Here's how the part is built. I have some questions about the finished solid (model axes, mm). A direction names the side the tool comes from. Coordinates: 2 decimals unless noted, no trailing zeros. Order: outer loops, then holes, each group sorted by start corner. A loop starts at its lowest first (then second) coordinate and runs counter-clockwise, first axis right, second up. Notation, with made-up numbers: M -29,34.5 L 29,34.5 A22 ccw 29,61.5 Z; hole C 53.25,75 d8. An arc over 180 degrees is marked long. Answer as CSV lines item,"result". Start each with the question number.
```python
from build123d import *

# Parameters (mm, degrees)
SKETCH1_W           = 82.042
SKETCH1_H           = 56.388
SKETCH1_R           = 1.651
BOSS_EXTRUDE1_DEPTH = 2.54
SKETCH2_W           = 19.05
SKETCH2_H           = 2.7432
SKETCH2_W_2         = 2.7432
SKETCH2_H_2         = 19.05
BOSS_EXTRUDE2_DEPTH = 2.54
SKETCH3_W           = 30.48
SKETCH3_H           = 9.525
CUT_EXTRUDE1_DEPTH  = 3.54


with BuildPart() as part:
    # Sketch1 → Boss-Extrude1 (new body)
    with BuildSketch(Plane(origin=(0, 0, 0), x_dir=(1, 0, 0), z_dir=(0, 1, 0))):
        Rectangle(SKETCH1_W, SKETCH1_H)
        with Locations((-34.671, 21.844)):
            Circle(SKETCH1_R, mode=Mode.SUBTRACT)
        with Locations((-34.671, -21.844)):
            Circle(SKETCH1_R, mode=Mode.SUBTRACT)
        with Locations((34.671, -21.844)):
            Circle(SKETCH1_R, mode=Mode.SUBTRACT)
        with Locations((34.671, 21.844)):
            Circle(SKETCH1_R, mode=Mode.SUBTRACT)
    extrude(amount=BOSS_EXTRUDE1_DEPTH)

    # Sketch2 → Boss-Extrude2 (add)
    with BuildSketch(Plane(origin=(0, 2.54, 0), x_dir=(1, 0, 0), z_dir=(0, 1, 0))):
        with Locations((0, 29.5656)):
            Rectangle(SKETCH2_W, SKETCH2_H)
        with Locations((0, -29.5656)):
            Rectangle(SKETCH2_W, SKETCH2_H)
        with Locations((42.3926, 0)):
            Rectangle(SKETCH2_W_2, SKETCH2_H_2)
        with Locations((-42.3926, 0)):
            Rectangle(SKETCH2_W_2, SKETCH2_H_2)
    extrude(amount=-BOSS_EXTRUDE2_DEPTH)

    # Sketch3 → Cut-Extrude1 (cut, through all)
    with BuildSketch(Plane(origin=(0, 2.54, 0), x_dir=(1, 0, 0), z_dir=(0, 1, 0))):
        with Locations((14.351, 21.5265)):
            Rectangle(SKETCH3_W, SKETCH3_H)
    extrude(amount=-CUT_EXTRUDE1_DEPTH, mode=Mode.SUBTRACT)


solid = part.part
```
1) I need wall thicknesses on line 1 (Z direction, x = -34.5, y = 1.4); line 2 (Z direction, x = 22, y = 2); line 3 (Z direction, x = 5, y = 2.1). Which ranges of each line are inside material? Lowest first, please. Write a range as [from, to].
2) Suppose I cut it at B-B on z = -19. Please give me the cut outline in (x, y), plus the area to 3 significant figures.
3) Suppose I cut it at D-D on x = 34.5. Please give me the cut outline in (y, z).
4) Suppose I cut it at C-C on y = 1.3. Please give me the cut outline in (x, z) (3 decimals), plus the area to 3 significant figures.
5) Suppose I cut it at A-A on x = 23. Please give me the cut outline in (y, z), plus the area to 3 significant figures.
6) Will these pins go through, and if not, where does the flat tip stop? pin 1 Ø0.8 at (x, y) = (42, 1) entering from +Z (3 decimals); pin 2 Ø3 at (x, z) = (34.671, -21.844) entering from -Y (3 decimals); pin 3 Ø0.8 at (y, z) = (1.5, -29) entering from -X (3 decimals); pin 4 Ø1 at (y, z) = (0.5, -12.5) entering from -X.
7) If we mould it in two halves opening along Z, with no side actions, what happens to faces 1 (the face through (42, 1, 9.525)), 2 (the face through (14, 1, -16.764)), 3 (the face through (-42, 1, -9.525)), 4 (the face through (14, 1, -26.289))? For each: released by +Z, released by -Z, zero draft, split by the parting line, or undercut.
8) Which directions (+Z, -Z, +X, -X, +Y, -Y) give clear straight access to the entire face, cutting with the end or side of a thin tool? Please do faces 5 (the face through (41.021, 1, 19)), 6 (the face through (-0.889, 1, -21)), 7 (the face through (-25, 1, 28.194)), 8 (the face through (9.525, 1, -30)).
Output:
1,line 1,"[-28.19, -23.49], [-20.2, 20.2], [23.49, 28.19]"
1,line 2,"[-28.19, -26.29], [-16.76, 28.19]"
1,line 3,"[-30.94, -26.29], [-16.76, 30.94]"
2,outline,"M -41.02,0 L -0.89,0 L -0.89,2.54 L -41.02,2.54 Z; M 29.59,0 L 41.02,0 L 41.02,2.54 L 29.59,2.54 Z"
2,area,"131 mm²"
3,outline,"M 0,-28.19 L 2.54,-28.19 L 2.54,-23.49 L 0,-23.49 Z; M 0,-20.2 L 2.54,-20.2 L 2.54,20.2 L 0,20.2 Z; M 0,23.49 L 2.54,23.49 L 2.54,28.19 L 0,28.19 Z"
4,outline,"M -43.764,-9.525 L -41.021,-9.525 L -41.021,-28.194 L -9.525,-28.194 L -9.525,-30.937 L 9.525,-30.937 L 9.525,-28.194 L 41.021,-28.194 L 41.021,-9.525 L 43.764,-9.525 L 43.764,9.525 L 41.021,9.525 L 41.021,28.194 L 9.525,28.194 L 9.525,30.937 L -9.525,30.937 L -9.525,28.194 L -41.021,28.194 L -41.021,9.525 L -43.764,9.525 Z; hole C -34.671,-21.844 d3.302; hole C -34.671,21.844 d3.302; hole M -0.889,-26.289 L 29.591,-26.289 L 29.591,-16.764 L -0.889,-16.764 Z; hole C 34.671,-21.844 d3.302; hole C 34.671,21.844 d3.302"
4,area,"4,510 mm²"
5,outline,"M 0,-28.19 L 2.54,-28.19 L 2.54,-26.29 L 0,-26.29 Z; M 0,-16.76 L 2.54,-16.76 L 2.54,28.19 L 0,28.19 Z"
5,area,"119 mm²"
6,pin 1,"z = 9.525"
6,pin 2,"through"
6,pin 3,"x = -9.525"
6,pin 4,"x = -41.02"
7,face 1,"released by +Z"
7,face 2,"undercut"
7,face 3,"released by -Z"
7,face 4,"undercut"
8,face 5,"+Z, +X, +Y, -Y"
8,face 6,"+Y, -Y"
8,face 7,"+Z, -X, +Y, -Y"
8,face 8,"-Z, +X, +Y, -Y"
